```python
from build123d import *

# Parameters (mm, degrees)
SKETCH2_R           = 2.5
SKETCH3_R           = 3.5
BOSS_EXTRUDE1_DEPTH = 2
SKETCH4_R           = 5
BOSS_EXTRUDE2_DEPTH = 6


with BuildPart() as part:
    # Sweep1: sweep along a path in Sketch1
    with BuildLine(Plane.XY) as sweep1_path:
        Line((0, 21), (0, 0))
        Line((0, 0), (15, 0))
    # Sketch2 → Sweep1 (sweep)
    with BuildSketch(Plane(origin=(15, 0, 0), x_dir=(0, 0, -1), z_dir=(1, 0, 0))):
        Circle(SKETCH2_R)
    sweep(path=sweep1_path.line, transition=Transition.RIGHT)

    # Sketch3 → Boss-Extrude1 (add)
    with BuildSketch(Plane(origin=(15, 0, 0), x_dir=(0, 0, -1), z_dir=(1, 0, 0))):
        Circle(SKETCH3_R)
    extrude(amount=BOSS_EXTRUDE1_DEPTH)

    # Sketch4 → Boss-Extrude2 (add)
    with BuildSketch(Plane(origin=(0, 21, 0), x_dir=(1, 0, 0), z_dir=(0, 1, 0))):
        with Locations(Location((0, 0, 0), (0, 0, 180))):
            Circle(SKETCH4_R)
    extrude(amount=BOSS_EXTRUDE2_DEPTH)


solid = part.part
```
Here's how the part is built. I have some questions about the finished solid (model axes, mm). A direction names the side the tool comes from. Coordinates: 2 decimals unless noted, no trailing zeros. Write each loop counter-clockwise with the first axis right and the second up, starting at its lowest first coordinate (ties: lowest second). Pieces come first, ordered by that corner, then holes. Notation, with made-up numbers: (-7, 32.25) -> (-2, 32.25) arc R21 ccw to (-2, 56.25) -> close; hole circle Ø6 at (71.5, -37.75). An arc over 180 degrees is marked (long way). Use a Markdown table: item, result. Add a question column.
(1) Please list where these lines run through material, in increasing order: line 1 (X direction, y = 4, z = 0); line 2 (X direction, y = 1, z = 0); line 3 (Z direction, x = -0.25, y = 23.5).
(2) If we section it at B-B, the plane y = 0: Write out the boundary of the cut face in (x, z), and give its area (3 significant figures).
(3) If we section it at A-A, the plane x = 3: Write out the boundary of the cut face in (y, z), and give its area (3 significant figures).
(4) We'd pull the mould along X, two halves only. Please class faces 4 (the cylindrical face through (5, 24, 0)), 5 (the flat face through (15, -2, -2)), 6 (the cylindrical face through (8.32, -2.44, 0.54)), 7 (the flat face through (-2, 21, -2)): +X half, -X half, draft (parallel to the pull), parting line (faces both ways), or undercut.
(5) If we section it at C-C, the plane x = 0: Write out the boundary of the cut face in (y, z), and give its area (3 significant figures).
(6) For faces 1 (the flat face through (17, 0, 0)), 2 (the cylindrical face through (15.986, -1.341, -3.233)), 3 (the cylindrical face through (-2.44, 9.09, 0.54)), which set-ups out of +Z, -Z, +X, -X, +Y, -Y let a thin tool reach every point of the face, with its end or its side?
(7) If we section it at D-D, the plane z = 0: Write out the boundary of the cut face in (x, y), and give its area (3 significant figures).
(8) I'm going to push flat-ended pins straight in: P1, Ø3.5, axis at y = 0, z = 0.5, coming from the -X side; P2, Ø2, axis at x = 10, z = -0.5, coming from the -Y side; P3, Ø4, axis at x = 3, z = -2.5, coming from the -Y side. Where does each tip first touch, or does it pass through?
Outcome:
| question | item | result |
|---|---|---|
| 1 | line 1 | x = -2.5 to 2.5 |
| 1 | line 2 | x = -2.5 to 17 |
| 1 | line 3 | z = -4.99 to 4.99 |
| 2 | outline | (0, -2.5) -> (15, -2.5) -> (15, -3.5) -> (17, -3.5) -> (17, 3.5) -> (15, 3.5) -> (15, 2.5) -> (0, 2.5) arc R2.5 ccw to start |
| 2 | area | 98.8 mm^2 |
| 3 | outline | circle Ø5 at (0, 0); (21, -4) -> (27, -4) -> (27, 4) -> (21, 4) -> close |
| 3 | area | 67.6 mm^2 |
| 4 | face 4 | parting line |
| 4 | face 5 | undercut |
| 4 | face 6 | undercut |
| 4 | face 7 | draft |
| 5 | outline | (0, -2.5) -> (21, -2.5) -> (21, -5) -> (27, -5) -> (27, 5) -> (21, 5) -> (21, 2.5) -> (0, 2.5) arc R2.5 ccw to start |
| 5 | area | 175 mm^2 |
| 6 | face 1 | +Z, -Z, +X, +Y, -Y |
| 6 | face 2 | +X |
| 6 | face 3 | none |
| 7 | outline | (-5, 21) -> (-2.5, 21) -> (-2.5, -2.5) -> (15, -2.5) -> (15, -3.5) -> (17, -3.5) -> (17, 3.5) -> (15, 3.5) -> (15, 2.5) -> (2.5, 2.5) -> (2.5, 21) -> (5, 21) -> (5, 27) -> (-5, 27) -> close |
| 7 | area | 254 mm^2 |
| 8 | P1 | stops at x = -2.5 |
| 8 | P2 | stops at y = -2.5 |
| 8 | P3 | stops at y = -2.45 |
